Model file for the job. Use its own axes, mm. Face numbers are marked on the shaded views. A direction names the side the tool comes from. Round coordinates to 2 decimals unless told otherwise and drop trailing zeros. Order: outer loops, then holes, each group sorted by start corner. A loop starts at its lowest first (then second) coordinate and runs counter-clockwise, first axis right, second up. Notation, with made-up numbers: (69.5, 3.25) - (83.5, 3.25) arc R14 cw to (83.5, 14.25) - close; hole circle Ø3 at (16, 48). An arc over 180 degrees is marked (long way). Put each result on its own line as item: value. Start each with the question number.
Item 1: Which spindle directions (+Z, -Z, +X, -X, +Y, -Y) get a long thin tool onto all of the face, cutting with end or side? Do the marked faces 4, 5 and 6. Say none if no direction does.
Item 2: Saw through at B-B on x = 46. List the corners of the cut face in (y, z).
Item 3: Probe probe 1 along Y at (x, z) = (12.7, 0); probe 2 along X at (y, z) = (-7, -11); probe 3 along X at (y, z) = (-4, -9). List the from-to ranges inside material, lowest first.
Item 4: Saw through at A-A on x = 22.5. List the corners of the cut face in (y, z), plus the area to 3 significant figures.
Item 5: Mould opens along Z. For the marked faces 1, 2 and 3 say: pulls with the +Z half, pulls with the -Z half, needs draft (parallel to the pull), parting line crosses it, or undercut.
Item 6: Pin check, flat tips, straight feed: pin 1 Ø4 at (y, z) = (-2, -6) entering from -X; pin 2 Ø2.5 at (y, z) = (3.5, -6.5) entering from -X; pin 3 Ø1 at (x, y) = (102.5, -8) entering from -Z. Stop position of each tip, or through.
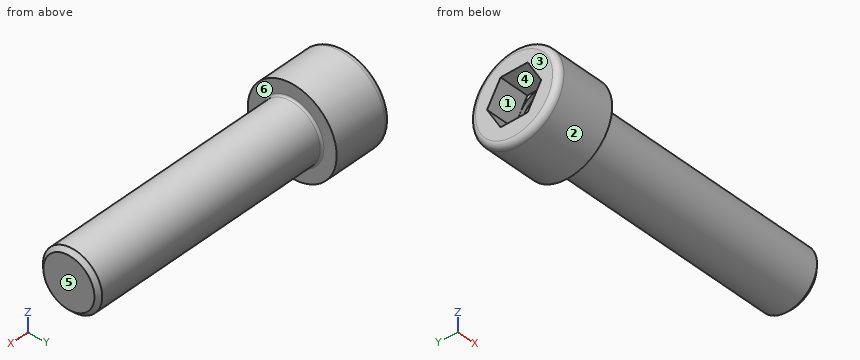
```python
from build123d import *

# Parameters (mm, degrees)
BASEHEADSKE_R   = 18
BASEHEAD_DEPTH  = 24
CUTSOCKET_DEPTH = 12
FILLET1_R       = 0.8
FILLET2_R       = 2.4


with BuildPart() as part:
    # BaseHeadSke → BaseHead (new body)
    with BuildSketch(Plane(origin=(0, 0, 0), x_dir=(0, 0, -1), z_dir=(1, 0, 0))):
        Circle(BASEHEADSKE_R)
    extrude(amount=BASEHEAD_DEPTH)

    # BodySke → BaseBody (revolve)
    with BuildSketch(Plane.XY):
        Polygon((0, 0), (124, 0), (124, 10.352), (122.352, 12), (0, 12), align=None)
    revolve(axis=Axis((0, 0, 0), (1, 0, 0)))

    # CutSocketSke → CutSocket (cut)
    with BuildSketch(Plane(origin=(0, 0, 0), x_dir=(0, 0, -1), z_dir=(1, 0, 0))):
        Polygon((0, 10.969655115), (-9.5, 5.484827557), (-9.5, -5.484827557), (0, -10.969655115), (9.5, -5.484827557), (9.5, 5.484827557), align=None)
    extrude(amount=CUTSOCKET_DEPTH, mode=Mode.SUBTRACT)

    # CutHoleSke → CutHole (revolve, cut)
    with BuildSketch(Plane.XY):
        Polygon((0, 9.5), (13.6, 9.5), (19.084827557, 0), (0, 0), align=None)
    revolve(axis=Axis((0, 0, 0), (1, 0, 0)), mode=Mode.SUBTRACT)

    # Fillet1
    fillet1_edges = [part.edges().sort_by_distance(p)[0] for p in [
        (24, -12, 0),
    ]]
    fillet(fillet1_edges, radius=FILLET1_R)

    # Fillet2
    fillet2_edges = [part.edges().sort_by_distance(p)[0] for p in [
        (0, 0, 18),
    ]]
    fillet(fillet2_edges, radius=FILLET2_R)


solid = part.part
```
Results found:
1. face 4: -X
1. face 5: +Z, -Z, +X, +Y, -Y
1. face 6: +X
2. outline: circle Ø24 at (0, 0)
3. probe 1: y = -18 to -9.5, 9.5 to 18
3. probe 2: x = 0 to 24
3. probe 3: x = 12 to 124
4. outline: circle Ø36 at (0, 0)
4. area: 1,020 mm²
5. face 1: undercut
5. face 2: parting line crosses it
5. face 3: needs draft
6. pin 1: stops at x = 14.28
6. pin 2: stops at x = 14.1
6. pin 3: stops at z = -9.37
